Verification items for the finished model (mm, model axes). A direction names the side the tool comes from. Coordinates: 2 decimals unless noted, no trailing zeros. Loops run counter-clockwise (first coordinate to the right, second up) from the corner with the lowest first, then second, coordinate; pieces in that order, holes last. Notation, with made-up numbers: (37, 71.25) -> (60, 71.25) arc R22 cw to (60, 95.25) -> close; hole circle Ø10 at (89.5, 12.25). An arc over 180 degrees is marked (long way). Write item = value, one per line.
```python
from build123d import *

# Parameters (mm, degrees)
SKETCH_1_W          = 20
SKETCH_1_H          = 20
SKETCH_1_W_2        = 16
SKETCH_1_H_2        = 16
EXTRUDE_1_DEPTH     = 275
SKETCH_3_R          = 2.5
CUT_EXTRUDE_2_DEPTH = 276.907593226
SKETCH_4_R          = 2.5
CUT_EXTRUDE_3_DEPTH = 276.907593226


with BuildPart() as part:
    # 草图1 → 凸台-拉伸1 (new body)
    with BuildSketch(Plane.XY):
        Rectangle(SKETCH_1_W, SKETCH_1_H)
        Rectangle(SKETCH_1_W_2, SKETCH_1_H_2, mode=Mode.SUBTRACT)
    extrude(amount=EXTRUDE_1_DEPTH)

    # 草图3 → 切除-拉伸2 (cut, through all)
    with BuildSketch(Plane.XZ.offset(10)):
        with Locations(Location((0, 7.5, 0), (0, 0, 270))):
            Circle(SKETCH_3_R)
        with Locations(Location((0, 267.5, 0), (0, 0, 180))):
            Circle(SKETCH_3_R)
        with Locations(Location((0, 22.5, 0), (0, 0, 180))):
            Circle(SKETCH_3_R)
        with Locations(Location((0, 252.5, 0), (0, 0, 270))):
            Circle(SKETCH_3_R)
    extrude(amount=-CUT_EXTRUDE_2_DEPTH, mode=Mode.SUBTRACT)

    # 草图4 → 切除-拉伸3 (cut, through all)
    with BuildSketch(Plane.ZY.offset(10)):
        with Locations(Location((107.5, 0, 0), (0, 0, 270))):
            Circle(SKETCH_4_R)
        with Locations(Location((167.5, 0, 0), (0, 0, 90))):
            Circle(SKETCH_4_R)
        with Locations(Location((137.5, 0, 0), (0, 0, 270))):
            Circle(SKETCH_4_R)
    extrude(amount=-CUT_EXTRUDE_3_DEPTH, mode=Mode.SUBTRACT)


solid = part.part
```
1) Material ranges on line 1 (Z direction, x = 9, y = 0.5); line 2 (Y direction, x = -2.5, z = 252); line 3 (X direction, y = 8.7, z = 7.5), recorded low to high.
Ans:
line_1 = 0 to 105.05, 109.95 to 135.05, 139.95 to 165.05, 169.95 to 275
line_2 = -10 to -8, 8 to 10
line_3 = -10 to -2.5, 2.5 to 10
2) Sectioned sample at C-C, the plane z = 267.5. Record the cut outline in (x, y), plus the area to 3 significant figures.
Ans:
outline = (-10, -10) -> (-2.5, -10) -> (-2.5, -8) -> (-8, -8) -> (-8, 8) -> (-2.5, 8) -> (-2.5, 10) -> (-10, 10) -> close; (2.5, -10) -> (10, -10) -> (10, 10) -> (2.5, 10) -> (2.5, 8) -> (8, 8) -> (8, -8) -> (2.5, -8) -> close
area = 124 mm2
3) Sectioned sample at A-A, the plane z = 221. Record the cut outline in (x, y).
Ans:
outline = (-10, -10) -> (10, -10) -> (10, 10) -> (-10, 10) -> close; hole (-8, -8) -> (8, -8) -> (8, 8) -> (-8, 8) -> close
4) Depth check by flat-ended pin: pin 1 Ø4.5 at (y, z) = (0, 107.5) entering from +X; pin 2 Ø5 at (x, y) = (-3.5, 6.5) entering from -Z. Enter the tip coordinate at first touch or a pass-through.
Ans:
pin_1 = through
pin_2 = 0
5) Sectioned sample at B-B, the plane y = 0. Count the separate pieces of the cut face and the enclosed holes in it, plus the area to 3 significant figures.
Ans:
separate_pieces = 8
enclosed_holes = 0
area = 1,040 mm2
6) Release check for a two-part mould opening along Y. For faces 1 (the face through (0, -10, 136)), 2 (the face through (10, -2.4, 135.6)), 3 (the face through (9, 0, 165)) record: pulls with the +Y half, pulls with the -Y half, needs draft (parallel to the pull), parting line crosses it, or undercut.
Ans:
face_1 = pulls with the -Y half
face_2 = needs draft
face_3 = undercut
7) Tool access check on faces 4 (the face through (-9, 0, 140)), 5 (the face through (0, 8, 136)). Record the directions out of +Z, -Z, +X, -X, +Y, -Y that give a thin tool (end or side, any length) a straight path to the whole face; none if there is none.
Ans:
face_4 = +X, -X
face_5 = +Z, -Z
